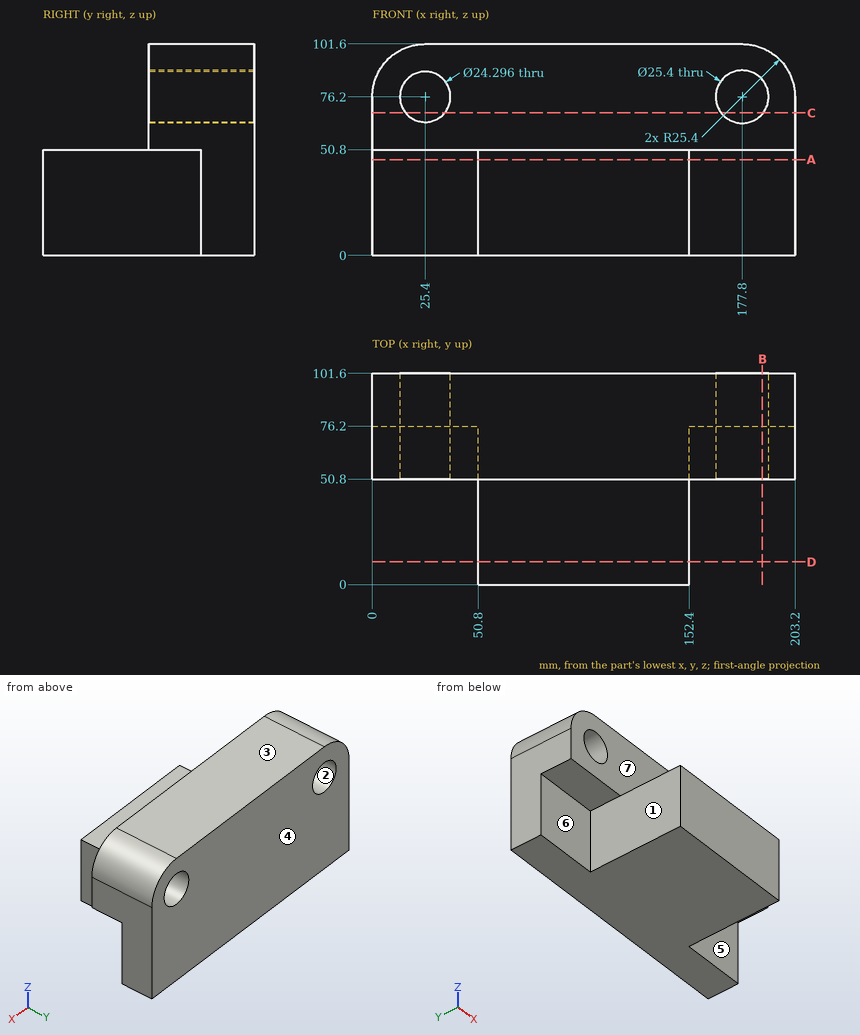
Geometry check sheet. Reference: drawing and pictorial views, mm from the part's lowest x, y, z. A direction names the side the tool comes from. Give positions to 0.01 mm unless a question says otherwise; leave off trailing zeros. Write each loop counter-clockwise with the first axis right and the second up, starting at its lowest first coordinate (ties: lowest second). Pieces come first, ordered by that corner, then holes. Notation, with made-up numbers: M 40,-12 L 80,-12 A11 ccw 80,2 Z; hole C -39,88.25 d11. An arc over 180 degrees is marked long. Answer as CSV lines item,"result". Start each with the question number.
Q1. Tool access check on the marked faces 4, 5, 6 and 7. Record the directions out of +Z, -Z, +X, -X, +Y, -Y that give a thin tool (end or side, any length) a straight path to the whole face; none if there is none.
Q2. Section check A-A, the plane z = 46. Record the cut outline in (x, y).
Q3. Section check B-B, the plane x = 187.5. Record the cut outline in (y, z) (1 decimal), then the cut area to 3 significant figures.
Q4. Section check C-C, the plane z = 68.5. Record the cut outline in (x, y) (1 decimal), then the cut area to 3 significant figures.
Q5. Release check for a two-part mould opening along X. For the marked faces 1, 2 and 3 record: pulls with the +X half, pulls with the -X half, needs draft (parallel to the pull), parting line crosses it, or undercut.
Q6. Go/stop test with flat-tipped pins: pin 1 (12.5 mm diameter, centred on x = 25, y = 67.5, fed in from -Z); pin 2 (15 mm diameter, centred on x = 116, y = 29, fed in from +Z); pin 3 (6 mm diameter, centred on x = 53.5, z = 68.5, fed in from -Y). Record where each tip stops, or that it passes through.
Q7. Material ranges on L1, parallel to X at y = 76, z = 76; L2, parallel to X at y = 57, z = 68.5 (1 decimal); L3, parallel to Z at x = 177.8, y = 91.5, recorded low to high.
Q8. Section check D-D, the plane y = 11. Record the cut outline in (x, z).
Geometry says:
1,face 4,"+Z, -Z, +X, -X, +Y"
1,face 5,"-Z, +X, -Y"
1,face 6,"-Z, -X, -Y"
1,face 7,"+Z, +X, -X, -Y"
2,outline,"M 0,76.2 L 50.8,76.2 L 50.8,0 L 152.4,0 L 152.4,76.2 L 203.2,76.2 L 203.2,101.6 L 0,101.6 Z"
3,outline,"M 50.8,50.8 L 76.2,50.8 L 76.2,0 L 101.6,0 L 101.6,68 L 50.8,68 Z; M 50.8,84.4 L 101.6,84.4 L 101.6,99.7 L 50.8,99.7 Z"
3,area,"2,940 mm^2"
4,outline,"M 0,50.8 L 16,50.8 L 16,101.6 L 0,101.6 Z; M 34.8,50.8 L 167.7,50.8 L 167.7,101.6 L 34.8,101.6 Z; M 187.9,50.8 L 203.2,50.8 L 203.2,101.6 L 187.9,101.6 Z"
4,area,"8,340 mm^2"
5,face 1,"pulls with the -X half"
5,face 2,"undercut"
5,face 3,"needs draft"
6,pin 1,"z = 50.8"
6,pin 2,"z = 50.8"
6,pin 3,"y = 50.8"
7,L1,"0 to 13.25, 37.55 to 165.1, 190.5 to 203.2"
7,L2,"0 to 16, 34.8 to 167.7, 187.9 to 203.2"
7,L3,"0 to 63.5, 88.9 to 101.6"
8,outline,"M 50.8,0 L 152.4,0 L 152.4,50.8 L 50.8,50.8 Z"
